Autodesk Inventor part; units mm, degrees
ref_plane "Slot Start Plane" through (0, 0, -1.7245) normal (0, 0, 1) x (1, 0, 0)
ref_plane "YZ Plane" through (0, 0, 0) normal (1, 0, 0) x (0, 1, 0)
ref_plane "XZ Plane" through (0, 0, 0) normal (0, 1, 0) x (-1, 0, 0)
ref_plane "Slot Start Plane" through (0, 0, -1.7245) normal (0, 0, 1) x (1, 0, 0)
sketch "Key Profile" plane through (0, 0, 0) normal (1, 0, 0) x (0, 1, 0)
  line L0 (-2, 2.8563) -> (0.684, 1.8794)
  arc A0 (1.6188, -1.1745) -> (0.684, 1.8794) centre (0, 0) ccw
  line L1 (-2, 1.3132) -> (0.1881, 0.5168)
  arc A1 (0, -0.55) -> (0.1881, 0.5168) centre (0, 0) ccw
  line L2 (-2, 2.8563) -> (-2, -0.55)
  line L3 (0, 0) -> (-2, 0) construction
  line L4 (0, -0.55) -> (-2, -0.55)
  line L5 (1.6188, -1.1745) -> (-0.097, -0.55)
  line L6 (6, -5.55) -> (6, 87.7952)
  line L7 (-2, 87.9773) -> (-2, 2.8563)
  arc A2 (6, 87.7952) -> (-2, 87.9773) centre (0, 0) ccw
  line L8 (-2, -0.55) -> (-2, -7.55)
  arc A3 (4, -7.55) -> (6, -5.55) centre (4, -5.55) ccw
  line L9 (-2, -7.55) -> (4, -7.55)
  arc A4 (6, 55.1747) -> (-2, 55.464) centre (0, 0) ccw
  arc A5 (-2, 2.8563) -> (-2, 83.2148) centre (-539.3737, 43.0355) ccw
  point P0 (-0.5, 43.0355)
  point P1 (-0.6441, 55.4963)
  dimension "my_hingeCutRad" = 0.55
  dimension "my_hingeDepth" = 2
  dimension "my_hingeRegCutRad" = 2
  dimension "keyLength" = 88
  dimension "my_KeyHeight" = 8
  dimension "d107" = 20
  dimension "d122" = 4
  dimension "slotOffset" = 1.1745
  dimension "my_backWidth" = 7
  dimension "d128" = 55.5
  dimension "d135" = 1.5
  dimension "d136" = 4.7625
extrude "Upper (u)" add sketch "Key Profile" along normal blind 6.7 and the other way blind 4.8929 contours A5 A4 L6 A3 L9 L8 L4 L5 A0 L0 | L0 A0 L5 L4 A1 L1 L2
extrude "Lower (d)" add sketch "Key Profile" along normal blind 15.1786 and the other way blind 4.8929 contours A5 L7 A2 L6 A4
extrude "Protrusion Cutout" cut sketch "Key Profile" along normal mid plane 4.5 contours L0 A0 L5 L4 A1 L1 L2
fillet "Front Fillet" radius 1.5 1 edges at (5.1429, 6, 87.7952)
sketch "Slot Sketch" plane through (0, 0, -1.7245) normal (0, 0, 1) x (1, 0, 0)
  line L0 (2.15, -2) -> (2.15, 1)
  line L1 (3.1, 4) -> (-3.1, 4)
  line L2 (-2.15, 1) -> (-2.15, -2)
  line L3 (-2.15, -2) -> (2.15, -2)
  line L4 (0, -2) -> (0, 4) construction
  line L5 (-3.1, 4) -> (-3.1, 1)
  line L6 (-3.1, 1) -> (-2.15, 1)
  line L7 (2.15, 1) -> (3.1, 1)
  line L8 (3.1, 1) -> (3.1, 4)
  point P0 (0, 0)
  dimension "d109" = 2
  dimension "my_slotHeadOffset" = 1
  dimension "my_slotHeadHeight" = 3
  dimension "my_slotHeadWidth" = 6.2
  dimension "my_neckSlotWidth" = 4.3
extrude "Slot" cut sketch "Slot Sketch" against normal through all
fillet "Edge Softening" radius 0.7 13 edges at (6.7, 5.4142, -6.9642) (6.7, 1, -7.55) (6.7, 6, 24.8124) (-4.8929, 5.4142, -6.9642) (-4.8929, 1, -7.55) (-4.8929, 6, 40.4164) (-4.8929, 5.5879, 87.4156) (-4.8929, 1.2899, 87.9905) (15.1786, 5.5879, 87.4156) (15.1786, 1.2899, 87.9905) (15.1786, 6, 70.7788) (15.1786, 2.6828, 55.4351) (10.9393, 6, 55.1747)
equation "\"my_headHeight\" = 3"
equation "\"my_headOffset\" = 1"
equation "\"whiteKeyWidth\" = 20.07143"
properties part number "FKey0"
Design review of the part built by this model. Coordinates are the model's own, in mm. A direction names the side the tool comes from. Coordinates: 2 decimals unless noted, no trailing zeros. Loops run counter-clockwise (first coordinate to the right, second up) from the corner with the lowest first, then second, coordinate; pieces in that order, holes last. Notation, with made-up numbers: (-38, 61) - (-1, 61) arc R23 cw to (-1, 97) - close; hole circle Ø8 at (89.5, 0). An arc over 180 degrees is marked (long way). Use CSV: the item, a comma, the result in double quotes. Start each with the question number.
1. For faces 1 (the flat face through (3.1, 2, -5)), 2 (the cylindrical face through (-0.031, 1.905, 0.61)), 3 (the flat face through (4, 1, -7.55)), list the 3-axis set-ups (+Z, -Z, +X, -X, +Y, -Y) from which the entire face can be reached by the end or side of a thin tool; tool diameter is ignored.
2. Add section A-A on x = 13. Give the boundary of the cut face in (y, z).
3. To check wall thickness, follow probe 1 along X at (y, z) = (1.25, 1); probe 2 along X at (y, z) = (1.75, 4.5); probe 3 along Y at (x, z) = (4.5, 36.5). State the ranges of each line that lie inside material, in increasing order.
4. Mouldability with a two-part tool opening along Z and no side actions: class faces 4 (the flat face through (4.44, -0.92, 0.92)), 5 (the flat face through (-3.59, -0.92, 0.92)), 6 (the cylindrical face through (5.3, 5.6, 87.4)), 7 (the flat face through (-2.15, 0, -5)) as released by +Z, released by -Z, zero draft, split by the parting line, or undercut.
5. Add section C-C on z = 7. Give the boundary of the cut face in (x, y).
6. Add section B-B on z = 44. Give the boundary of the cut face in (x, y), plus the area to 3 significant figures.
7. Clearance check with flat-ended pins moving along their axes: pin 1 (0.6 mm diameter, centred on x = -2, y = -1.5, fed in from +Z); pin 2 (3.5 mm diameter, centred on y = -0.5, z = -3, fed in from +X); pin 3 (1.5 mm diameter, centred on x = 7, y = 0, fed in from -Z); pin 4 (5 mm diameter, centred on x = 11, z = 20.5, fed in from +Y). State where each tip first meets the part, or that it passes through.
Resolved:
1,face 1,"-Z"
1,face 2,"none"
1,face 3,"-Z, +X, -X, +Y, -Y"
2,outline,"(-2, 83.21) arc R538.88 cw to (-0.64, 55.5) arc R55.51 cw to (5.23, 55.25) arc R0.7 ccw to (6, 55.95) - (6, 86.38) arc R1.5 ccw to (4.58, 87.88) arc R88.02 ccw to (-2, 87.98) - close"
3,probe 1,"-4.89 to -2.25, 2.25 to 6.7"
3,probe 2,"-4.89 to 6.7"
3,probe 3,"-0.54 to 6"
4,face 4,"undercut"
4,face 5,"undercut"
4,face 6,"released by +Z"
4,face 7,"zero draft"
5,outline,"(-4.89, -1.71) - (6.7, -1.71) - (6.7, 5.3) arc R0.7 ccw to (6, 6) - (-4.19, 6) arc R0.7 ccw to (-4.89, 5.3) - close"
6,outline,"(-4.89, -0.5) - (6.7, -0.5) - (6.7, 5.3) arc R0.7 ccw to (6, 6) - (-4.19, 6) arc R0.7 ccw to (-4.89, 5.3) - close"
6,area,"75.2 mm2"
7,pin 1,"z = 87.99"
7,pin 2,"x = 6.7"
7,pin 3,"z = -7.5"
7,pin 4,"through"
